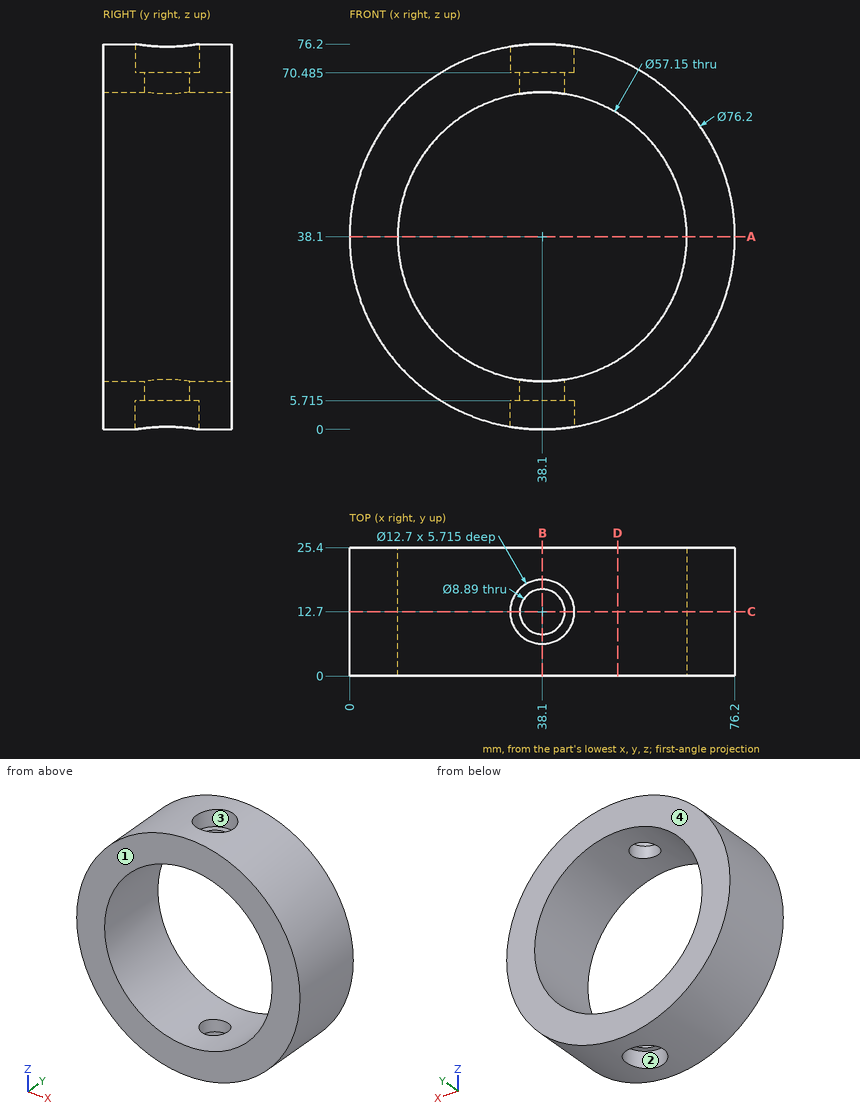
Can you work these out from the drawing? Everything is in mm from the part's minimum corner. Give positions to 0.01 mm unless a question says otherwise; leave off trailing zeros. Write each loop counter-clockwise with the first axis right and the second up, starting at its lowest first coordinate (ties: lowest second). Pieces come first, ordered by that corner, then holes. Notation, with made-up numbers: (13.5, 14) -> (23.5, 14) arc R23 cw to (23.5, 51) -> close; hole circle Ø1 at (-38, 50.25). An arc over 180 degrees is marked (long way). Write each question's results on one line, items separated by ' | '.
Item 1: Suppose I cut it at A-A on z = 38.1. Write out the boundary of the cut face in (x, y) (3 decimals), plus the area to 3 significant figures.
Output:
outline: (0, 0) -> (9.525, 0) -> (9.525, 25.4) -> (0, 25.4) -> close; (66.675, 0) -> (76.2, 0) -> (76.2, 25.4) -> (66.675, 25.4) -> close | area: 484 mm^2
Item 2: For pin 1 Ø10 at (x, y) = (38.1, 12.7) entering from -Z (3 decimals); pin 2 Ø12 at (x, y) = (58, 7) entering from -Z; pin 3 Ø6 at (x, y) = (55, 3.5) entering from +Z; pin 4 Ø8 at (x, z) = (17, 35) entering from -Y, each with a flat end and sliding along its axis, tell me the tip position at first contact or that it passes through.
Output:
pin 1: stops at z = 5.715 | pin 2: stops at z = 2.63 | pin 3: stops at z = 73.57 | pin 4: passes through
Item 3: Suppose I cut it at D-D on x = 53. Write out the boundary of the cut face in (y, z).
Output:
outline: (0, 3.03) -> (25.4, 3.03) -> (25.4, 13.72) -> (0, 13.72) -> close; (0, 62.48) -> (25.4, 62.48) -> (25.4, 73.17) -> (0, 73.17) -> close
Item 4: We'd pull the mould along Y, two halves only. Please class the marked faces 1, 2, 3 and 4: pulls with the +Y half, pulls with the -Y half, needs draft (parallel to the pull), parting line crosses it, or undercut.
Output:
face 1: pulls with the -Y half | face 2: undercut | face 3: undercut | face 4: pulls with the +Y half
Item 5: Suppose I cut it at B-B on x = 38.1. Write out the boundary of the cut face in (y, z) (3 decimals).
Output:
outline: (0, 0) -> (6.35, 0) -> (6.35, 5.715) -> (8.255, 5.715) -> (8.255, 9.525) -> (0, 9.525) -> close; (0, 66.675) -> (8.255, 66.675) -> (8.255, 70.485) -> (6.35, 70.485) -> (6.35, 76.2) -> (0, 76.2) -> close; (17.145, 5.715) -> (19.05, 5.715) -> (19.05, 0) -> (25.4, 0) -> (25.4, 9.525) -> (17.145, 9.525) -> close; (17.145, 66.675) -> (25.4, 66.675) -> (25.4, 76.2) -> (19.05, 76.2) -> (19.05, 70.485) -> (17.145, 70.485) -> close
Item 6: If I drill on L1, parallel to Y at x = 38.1, z = 74.65; L2, parallel to Y at x = 38, z = 67; L3, parallel to Z at x = 44.5, y = 2.25, over which ranges is the centre line in solid material (lowest first)?
Output:
L1: y = 0 to 6.35, 19.05 to 25.4 | L2: y = 0 to 8.26, 17.14 to 25.4 | L3: z = 0.54 to 10.25, 65.95 to 75.66
Item 7: Suppose I cut it at C-C on y = 12.7. Write out the boundary of the cut face in (x, z) (3 decimals), plus the area to 3 significant figures.
Output:
outline: (31.75, 0.533) -> (31.75, 5.715) -> (33.655, 5.715) -> (33.655, 9.873) arc R28.575 cw to (33.655, 66.327) -> (33.655, 70.485) -> (31.75, 70.485) -> (31.75, 75.667) arc R38.1 ccw to start; (42.545, 5.715) -> (44.45, 5.715) -> (44.45, 0.533) arc R38.1 ccw to (44.45, 75.667) -> (44.45, 70.485) -> (42.545, 70.485) -> (42.545, 66.327) arc R28.575 cw to (42.545, 9.873) -> close | area: 1,780 mm^2
